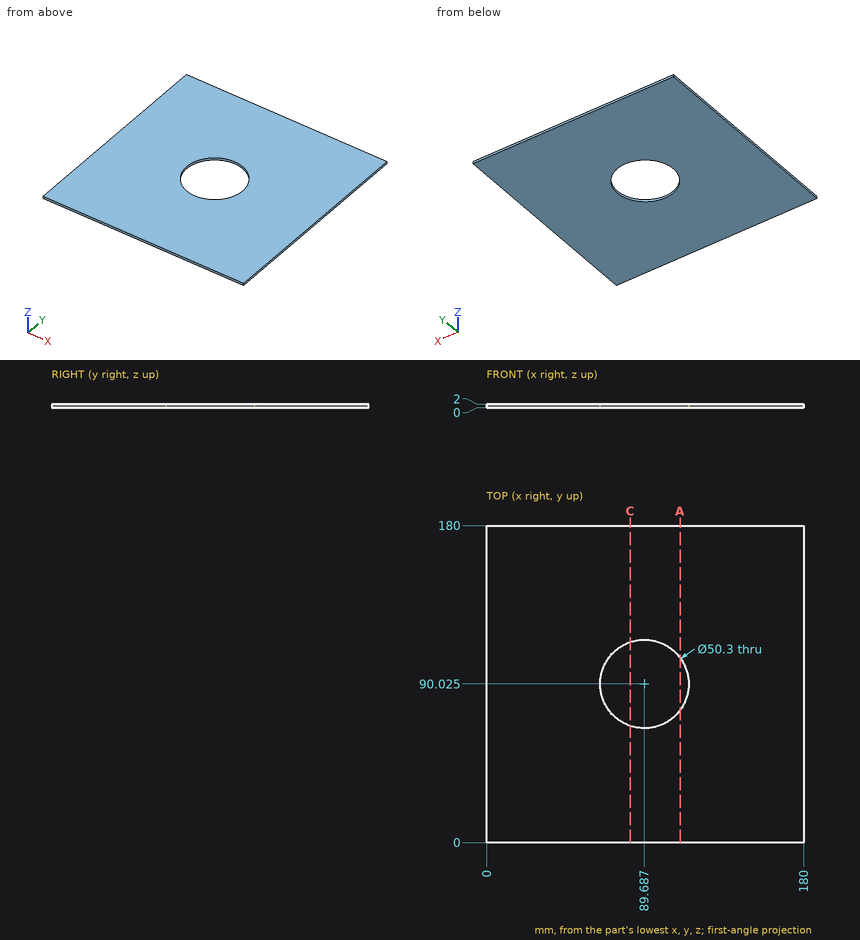
Can you work these out from the drawing? Everything is in mm from the part's minimum corner. Coordinates: 2 decimals unless noted, no trailing zeros. Write each loop counter-clockwise with the first axis right and the second up, starting at its lowest first coordinate (ties: lowest second). Pieces come first, ordered by that corner, then holes. Notation, with made-up numbers: (49.25, -24.75) - (88.25, -24.75) arc R27 ccw to (88.25, 0.25) - close; hole circle Ø10 at (33, 70). An arc over 180 degrees is marked (long way). Use a Markdown table: item, result.
Q1. Imagine slicing it at C-C (x = 81.5). List the corners of the cut face in (y, z) for me (1 decimal).
Geometry check:
| item | result |
|---|---|
| outline | (0, 0) - (66.2, 0) - (66.2, 2) - (0, 2) - close; (113.8, 0) - (180, 0) - (180, 2) - (113.8, 2) - close |
Q2. Imagine slicing it at A-A (x = 110). List the corners of the cut face in (y, z) for me (1 decimal).
Geometry check:
| item | result |
|---|---|
| outline | (0, 0) - (75.2, 0) - (75.2, 2) - (0, 2) - close; (104.9, 0) - (180, 0) - (180, 2) - (104.9, 2) - close |
Q3. Please list where these lines run through material, in increasing order: L1, parallel to X at y = 91, z = 1; L2, parallel to Y at x = 101, z = 1.8 (1 decimal); L3, parallel to X at y = 111, z = 1.6 (1 decimal).
Geometry check:
| item | result |
|---|---|
| L1 | x = 0 to 64.56, 114.82 to 180 |
| L2 | y = 0 to 67.6, 112.5 to 180 |
| L3 | x = 0 to 75.8, 103.6 to 180 |
